Geometry: see drawing. Coordinates: mm, zero at the bounding-box minimum. A direction names the side the tool comes from. Round coordinates to 2 decimals unless told otherwise and drop trailing zeros. Order: outer loops, then holes, each group sorted by start corner. A loop starts at its lowest first (then second) coordinate and runs counter-clockwise, first axis right, second up. Notation, with made-up numbers: (16.25, 13.5) -> (71.25, 13.5) arc R3 cw to (71.25, 18.5) -> close; hole circle Ø8 at (-1, -12). An arc over 180 degrees is marked (long way). Use a Markdown table: item, result.
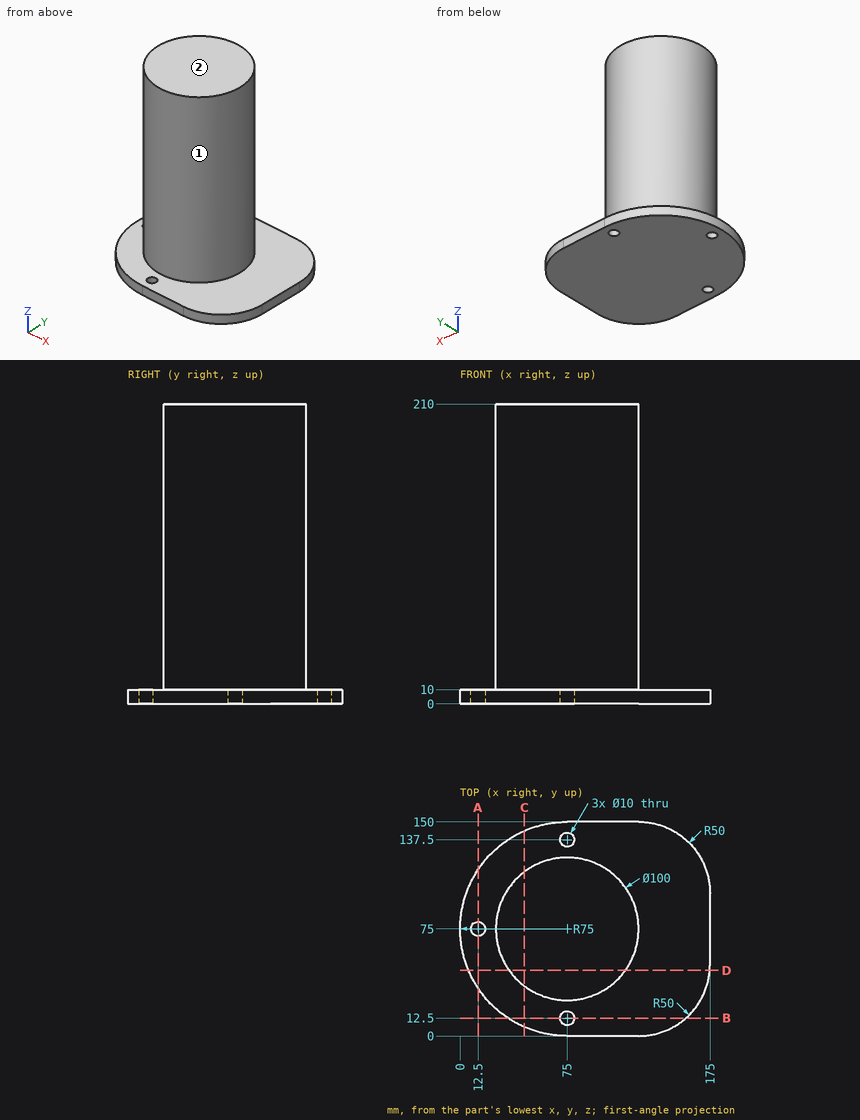
1) Cut plane A-A on x = 12.5. Return loops of the section in (y, z).
Answer key:
| item | result |
|---|---|
| outline | (33.54, 0) -> (70, 0) -> (70, 10) -> (33.54, 10) -> close; (80, 0) -> (116.46, 0) -> (116.46, 10) -> (80, 10) -> close |
2) Contact query for flat-ended pins moving along their axis: P1, Ø16, axis at x = 75, y = 12.5, coming from the +Z side; P2, Ø1.5, axis at y = 119.5, z = 167.5, coming from the -X side; P3, Ø6, axis at x = 40, z = 73, coming from the +Y side; P4, Ø6, axis at x = 12.5, y = 75, coming from the -Z side. Output: stop coordinate, or through.
Answer key:
| item | result |
|---|---|
| P1 | stops at z = 10 |
| P2 | stops at x = 50.79 |
| P3 | stops at y = 113.42 |
| P4 | passes through |
3) Ray query, probe 1 along Y at (x, z) = (75, 7); probe 2 along Z at (x, y) = (37, 16.5); probe 3 along Y at (x, z) = (12.5, 5.5). Return the intervals inside material, ascending.
Answer key:
| item | result |
|---|---|
| probe 1 | y = 0 to 7.5, 17.5 to 132.5, 142.5 to 150 |
| probe 2 | z = 0 to 10 |
| probe 3 | y = 33.54 to 70, 80 to 116.46 |
4) Cut plane C-C on x = 45. Return loops of the section in (y, z).
Answer key:
| item | result |
|---|---|
| outline | (6.26, 0) -> (143.74, 0) -> (143.74, 10) -> (115, 10) -> (115, 210) -> (35, 210) -> (35, 10) -> (6.26, 10) -> close |
5) Cut plane D-D on y = 46. Return loops of the section in (x, z), and give its area (3 significant figures).
Answer key:
| item | result |
|---|---|
| outline | (5.83, 0) -> (174.84, 0) -> (174.84, 10) -> (115.73, 10) -> (115.73, 210) -> (34.27, 210) -> (34.27, 10) -> (5.83, 10) -> close |
| area | 18,000 mm^2 |
6) Cut plane B-B on y = 12.5. Return loops of the section in (x, z), and give its area (3 significant figures).
Answer key:
| item | result |
|---|---|
| outline | (33.54, 0) -> (70, 0) -> (70, 10) -> (33.54, 10) -> close; (80, 0) -> (158.07, 0) -> (158.07, 10) -> (80, 10) -> close |
| area | 1,150 mm^2 |
7) Set-up query: the marked faces 1 and 2. Return all of +Z, -Z, +X, -X, +Y, -Y with unobstructed straight access to the full face (end or side cutting, diameter ignored); none if empty.
Answer key:
| item | result |
|---|---|
| face 1 | +Z |
| face 2 | +Z, +X, -X, +Y, -Y |
